```python
from build123d import *

# Parameters (mm, degrees)
SKETCH1_R           = 4
SKETCH1_R_2         = 4.198873956
BOSS_EXTRUDE1_DEPTH = 5
SKETCH2_R           = 13.5
BOSS_EXTRUDE2_DEPTH = 106
BOSS_EXTRUDE4_DEPTH = 4
CUT_EXTRUDE1_START  = -10
CUT_EXTRUDE1_DEPTH  = 10


with BuildPart() as part:
    # Sketch1 → Boss-Extrude1 (new body)
    with BuildSketch(Plane.XY.offset(32.670544835)):
        with BuildLine():
            Line((-70.496842865, 21.117824566), (-77.080259334, 45.687469315))
            Line((-77.080259334, 45.687469315), (29.171581558, 74.157564276))
            Line((29.171581558, 74.157564276), (32.157340999, 63.014558343))
            Line((32.157340999, 63.014558343), (-11.6122935, 35.626592223))
            ThreePointArc((-11.6122935, 35.626592223), (-40.615747818, 38.096615543), (-64.259394629, 21.117824566))
            Line((-64.259394629, 21.117824566), (-70.496842865, 21.117824566))
        make_face()
        with Locations((-65.433540443, 28.621355152)):
            Circle(SKETCH1_R, mode=Mode.SUBTRACT)
        with Locations((-51.195341682, 39.839935825)):
            Circle(SKETCH1_R, mode=Mode.SUBTRACT)
        with Locations((-33.791359384, 44.907899562)):
            Circle(SKETCH1_R, mode=Mode.SUBTRACT)
        with Locations((-15.756175362, 43.087187195)):
            Circle(SKETCH1_R_2, mode=Mode.SUBTRACT)
    extrude(amount=BOSS_EXTRUDE1_DEPTH)

    # Sketch2 → Boss-Extrude2 (add)
    with BuildSketch(Plane(origin=(-60.494993695, -16.209584707, 0), x_dir=(0, 0, 1), z_dir=(-0.9659258262890686, -0.2588190451025196, 0))):
        with BuildLine():
            Line((37.670544835, 64.080545666), (37.670544835, 64.282169128))
            ThreePointArc((37.670544835, 64.282169128), (35.170544835, 95.280545666), (32.670544835, 64.282169128))
            Line((32.670544835, 64.282169128), (32.670544835, 64.080545666))
            Line((32.670544835, 64.080545666), (37.670544835, 64.080545666))
        make_face()
        with Locations(Location((35.170544835, 79.680545666, 0), (0, 0, 270))):
            Circle(SKETCH2_R, mode=Mode.SUBTRACT)
    extrude(amount=-BOSS_EXTRUDE2_DEPTH)

    # Sketch3 → Boss-Extrude4 (add)
    with BuildSketch(Plane(origin=(41.893143892, 11.225234074, 0), x_dir=(0, 0, -1), z_dir=(0.9659258262890686, 0.2588190451025196, 0))):
        with BuildLine():
            Line((-37.670544835, 64.282169128), (-37.670544835, 64.080545666))
            Line((-37.670544835, 64.080545666), (-32.670544835, 64.080545666))
            Line((-32.670544835, 64.080545666), (-32.670544835, 64.282169128))
            ThreePointArc((-32.670544835, 64.282169128), (-35.170544835, 95.280545666), (-37.670544835, 64.282169128))
        make_face()
    extrude(amount=BOSS_EXTRUDE4_DEPTH)

    # Sketch4 → Cut-Extrude1 (cut)
    with BuildSketch(Plane.XY.offset(37.670544835).offset(CUT_EXTRUDE1_START)):
        with BuildLine():
            Line((-73.814643096, 33.500023595), (-49.675245154, 34.41948085))
            ThreePointArc((-49.675245154, 34.41948085), (-57.759852218, 28.637597873), (-64.259394629, 21.117824566))
            Line((-64.259394629, 21.117824566), (-70.496842865, 21.117824566))
            Line((-70.496842865, 21.117824566), (-73.814643096, 33.500023595))
        make_face()
    extrude(amount=CUT_EXTRUDE1_DEPTH, mode=Mode.SUBTRACT)


solid = part.part
```
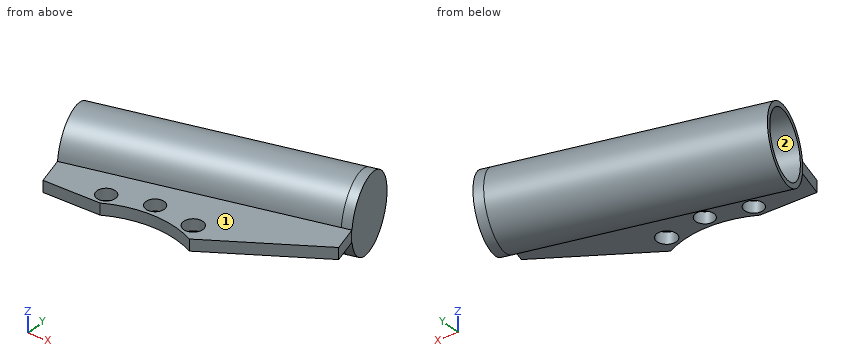
CAD build for the part. Positions are in the model's coordinates, mm. Face numbers are marked on the shaded views. Round coordinates to 2 decimals unless told otherwise and drop trailing zeros. Order: outer loops, then holes, each group sorted by start corner. A loop starts at its lowest first (then second) coordinate and runs counter-clockwise, first axis right, second up.
Q1. Slice it at C-C (z = 23.5). Write the cut outline in (x, y), and give its area (3 significant figures).
Q2. Drop flat-ended pins along their axis: pin 1 (1 mm diameter, centred on y = 77, z = 33, fed in from +X); pin 2 (10 mm diameter, centred on x = -9.5, z = 28.5, fed in from +Y); pin 3 (0.6 mm diameter, centred on x = 27.5, y = 73.5, fed in from -Z); pin 4 (6.5 mm diameter, centred on x = -33.79, y = 44.91, fed in from +Z). Give the stop position or say it passes through.
Q3. Slice it at B-B (x = -51). State how many separate pieces and enclosed holes the cut face has, and give its area (3 significant figures).
Q4. Two-plate mould, pull along Z, no slides. Class the marked faces 1 and 2: pulls with the +Z half, pulls with the -Z half, needs draft (parallel to the pull), parting line crosses it, or undercut.
Q5. Wall check: L1, parallel to Z at x = -49, y = 69.5; L2, parallel to Y at x = -35, z = 34.5; L3, parallel to Z at x = 8, y = 94. Give the ranges that are in metal, low to high.
Q6. Slice it at A-A (z = 41). Write the cut outline in (x, y).
Results below:
1. outline: (-83.8, 70.75) - (-82.87, 67.31) - (19.51, 94.75) - (23.03, 81.64) - (-79.36, 54.2) - (-78.44, 50.76) - (27.81, 79.23) - (22.45, 99.23) - close
1. area: 839 mm2
2. pin 1: stops at x = 28.54
2. pin 2: stops at y = 96.72
2. pin 3: stops at z = 32.67
2. pin 4: passes through
3. separate pieces: 2
3. enclosed holes: 1
3. area: 251 mm2
4. face 1: pulls with the +Z half
4. face 2: undercut
5. L1: z = 19.57 to 21.67, 48.67 to 50.77
5. L2: y = 39.24 to 41.09, 48.72 to 59.15, 87.07 to 89.25
5. L3: z = 22.46 to 25.15, 45.19 to 47.88
6. outline: (-84.86, 74.73) - (-84.27, 72.52) - (18.12, 99.95) - (24.42, 76.43) - (-77.97, 48.99) - (-77.37, 46.78) - (28.88, 75.25) - (21.39, 103.2) - close
